Read the model definition and answer for the solid it produces. Units are mm, in the model's axes. Coordinates: 2 decimals unless noted, no trailing zeros. Loops run counter-clockwise (first coordinate to the right, second up) from the corner with the lowest first, then second, coordinate; pieces in that order, holes last. Notation, with made-up numbers: (84, 72) -> (93, 72) arc R12 cw to (93, 95) -> close; hole circle Ø9 at (-38, 60.5). An arc over 180 degrees is marked (long way). Answer as a JSON object with one key per item and string values. Group by question number.
Q1. Determine the mould class of faces 1 (the cylindrical face through (82.63, 86.76, 11.71)), 2 (the flat face through (-2, -105, 12)), 3 (the flat face through (127, -1, 12)) for opening direction X: released by +X, released by -X, zero draft, split by the parting line, or undercut.
Q2. The part is cut by section A-A on y = 0. Write down the section's boundary in (x, z).
Q3. Straight lines are drawn through the part: line 1 along X through (y, z) = (-80, 18.75); line 2 along Y through (x, z) = (-90, 6.75); line 3 along X through (y, z) = (-88.5, 15.75). For each, find the intervals that lie inside material, in ascending order. Write a range as [from, to].
Q4. The part is cut by section D-D on z = 18. Write down the section's boundary in (x, y).
Q5. The part is cut by section C-C on x = -50. Write down the section's boundary in (y, z), and give its area (3 significant figures).
Q6. The part is cut by section B-B on x = 90. Write down the section's boundary in (y, z).
from build123d import *

# Parameters (mm, degrees)
SKETCH1_W           = 254
SKETCH1_H           = 210
SKETCH1_R           = 10
BOSS_EXTRUDE1_DEPTH = 25
CUT_EXTRUDE1_REACH  = 168.67
SKETCH2_R           = 10


with BuildPart() as part:
    # Sketch1 → Boss-Extrude1 (new body)
    with BuildSketch(Plane.XY):
        Rectangle(SKETCH1_W, SKETCH1_H)
        with Locations((-90, 80)):
            Circle(SKETCH1_R, mode=Mode.SUBTRACT)
        with Locations((90, 80)):
            Circle(SKETCH1_R, mode=Mode.SUBTRACT)
        with Locations((90, -80)):
            Circle(SKETCH1_R, mode=Mode.SUBTRACT)
        with Locations((-90, -80)):
            Circle(SKETCH1_R, mode=Mode.SUBTRACT)
    extrude(amount=BOSS_EXTRUDE1_DEPTH)

    # Sketch2 → Cut-Extrude1 (cut, up to next)
    with BuildSketch(Plane.XY.offset(25), mode=Mode.PRIVATE) as cut_extrude1_sk1:
        with Locations((-50, 0)):
            Circle(SKETCH2_R)
    cut_extrude1_tool1 = extrude(cut_extrude1_sk1.sketch, amount=-CUT_EXTRUDE1_REACH, mode=Mode.PRIVATE) & part.part
    # Sketch2 → Cut-Extrude1 (cut, up to next)
    with BuildSketch(Plane.XY.offset(25), mode=Mode.PRIVATE) as cut_extrude1_sk2:
        with Locations((50, 0)):
            Circle(SKETCH2_R)
    cut_extrude1_tool2 = extrude(cut_extrude1_sk2.sketch, amount=-CUT_EXTRUDE1_REACH, mode=Mode.PRIVATE) & part.part
    add(cut_extrude1_tool1.solids().sort_by_distance((-50, 0, 25))[0], mode=Mode.SUBTRACT)
    add(cut_extrude1_tool2.solids().sort_by_distance((50, 0, 25))[0], mode=Mode.SUBTRACT)

    # Cut-Extrude2 cone 1 section (through the dimple's axis) → Cut-Extrude2 (revolve, cut)
    with BuildSketch(Plane(origin=(-90, 80, 25), x_dir=(0, -1, 0), z_dir=(1, 0, 0))):
        Polygon((0, 0), (11.25, 0), (0, 11.25), align=None)
    revolve(axis=Axis((-90, 80, 25), (0, 0, -1)), mode=Mode.SUBTRACT)

    # Cut-Extrude2 cone 2 section (through the dimple's axis) → Cut-Extrude2 cone 2 (revolve, cut)
    with BuildSketch(Plane(origin=(90, 80, 25), x_dir=(0, -1, 0), z_dir=(1, 0, 0))):
        Polygon((0, 0), (11.25, 0), (0, 11.25), align=None)
    revolve(axis=Axis((90, 80, 25), (0, 0, -1)), mode=Mode.SUBTRACT)

    # Cut-Extrude2 cone 3 section (through the dimple's axis) → Cut-Extrude2 cone 3 (revolve, cut)
    with BuildSketch(Plane(origin=(90, -80, 25), x_dir=(0, -1, 0), z_dir=(1, 0, 0))):
        Polygon((0, 0), (11.25, 0), (0, 11.25), align=None)
    revolve(axis=Axis((90, -80, 25), (0, 0, -1)), mode=Mode.SUBTRACT)

    # Cut-Extrude2 cone 4 section (through the dimple's axis) → Cut-Extrude2 cone 4 (revolve, cut)
    with BuildSketch(Plane(origin=(-90, -80, 25), x_dir=(0, -1, 0), z_dir=(1, 0, 0))):
        Polygon((0, 0), (11.25, 0), (0, 11.25), align=None)
    revolve(axis=Axis((-90, -80, 25), (0, 0, -1)), mode=Mode.SUBTRACT)


solid = part.part
Final values:
{
 "1": {"face 1": "undercut", "face 2": "zero draft", "face 3": "released by +X"},
 "2": {"outline": "(-127, 0) -> (-60, 0) -> (-60, 25) -> (-127, 25) -> close; (-40, 0) -> (40, 0) -> (40, 25) -> (-40, 25) -> close; (60, 0) -> (127, 0) -> (127, 25) -> (60, 25) -> close"},
 "3": {"line 1": "x = [-127, -100], [-80, 80], [100, 127]", "line 2": "y = [-105, -90], [-70, 70], [90, 105]", "line 3": "x = [-127, -95.27], [-84.73, 84.73], [95.27, 127]"},
 "4": {"outline": "(-127, -105) -> (127, -105) -> (127, 105) -> (-127, 105) -> close; hole circle Ø20 at (-90, -80); hole circle Ø20 at (-90, 80); hole circle Ø20 at (-50, 0); hole circle Ø20 at (50, 0); hole circle Ø20 at (90, -80); hole circle Ø20 at (90, 80)"},
 "5": {"outline": "(-105, 0) -> (-10, 0) -> (-10, 25) -> (-105, 25) -> close; (10, 0) -> (105, 0) -> (105, 25) -> (10, 25) -> close", "area": "4,750 mm2"},
 "6": {"outline": "(-105, 0) -> (-90, 0) -> (-90, 23.75) -> (-91.25, 25) -> (-105, 25) -> close; (-70, 0) -> (70, 0) -> (70, 23.75) -> (68.75, 25) -> (-68.75, 25) -> (-70, 23.75) -> close; (90, 0) -> (105, 0) -> (105, 25) -> (91.25, 25) -> (90, 23.75) -> close"}
}
